The listing builds one solid part. Answer for the finished solid, in the listing's coordinates (mm). A direction names the side the tool comes from. Round coordinates to 2 decimals unless told otherwise and drop trailing zeros. Write each loop counter-clockwise with the first axis right and the second up, starting at its lowest first coordinate (ties: lowest second). Pieces come first, ordered by that corner, then holes.
(1) For faces 1 (the face through (18, 5, -0.1)), 2 (the face through (18, 0.808, -1)), 3 (the face through (18, 26, -2.4)), determine the directions among +Z, -Z, +X, -X, +Y, -Y from which every point of the face is accessible in a straight line to the end or side of a thin tool.
(2) Each of these flat-tipped pins is pushed along its axis until it touches: pin 1 Ø1.2 at (x, z) = (16, -1.5) entering from -Y; pin 2 Ø1.6 at (x, y) = (17, 4.5) entering from +Z. Where does it stop, or does it pass through?
(3) Find the intervals of material crossed by probe 1 along Y at (x, z) = (14, -1); probe 2 along Z at (x, y) = (29, 6), in increasing order.
(4) A cutting plane is placed at A-A, the plane x = 24. Give the vertices of the cut face in (y, z), and give its area (3 significant figures).
from build123d import *

# Parameters (mm, degrees)
ESQUISSE6_W             = 35.7
ESQUISSE6_H             = 51.2
BOSS_EXTRU_3_DEPTH      = 2.4
ESQUISSE7_W             = 33.59337029
ESQUISSE7_H             = 41.85
ENL_V_MAT_EXTRU_4_DEPTH = 0.1
ESQUISSE8_W             = 6.352818378
ESQUISSE8_H             = 0.449413723
ENL_V_MAT_EXTRU_5_DEPTH = 0.1
ESQUISSE9_W             = 31.478034176
ESQUISSE9_H             = 39.75
BOSS_EXTRU_4_DEPTH      = 0.1
ESQUISSE10_W            = 33.373849312
ESQUISSE10_H            = 5.346626879
ENL_V_MAT_EXTRU_6_DEPTH = 0.1
ESQUISSE11_W            = 23.638967436
ESQUISSE11_H            = 0.807997654
ENL_V_MAT_EXTRU_7_DEPTH = 63.463509347


with BuildPart() as part:
    # Esquisse6 → Boss.-Extru.3 (new body)
    with BuildSketch(Plane.XY):
        with Locations((17.85, 25.6)):
            Rectangle(ESQUISSE6_W, ESQUISSE6_H)
    extrude(amount=-BOSS_EXTRU_3_DEPTH)

    # Esquisse7 → Enlèv. mat.-Extru.4 (cut)
    with BuildSketch(Plane.XY):
        with Locations((17.85, 29.225)):
            Rectangle(ESQUISSE7_W, ESQUISSE7_H)
    extrude(amount=-ENL_V_MAT_EXTRU_4_DEPTH, mode=Mode.SUBTRACT)

    # Esquisse8 → Enlèv. mat.-Extru.5 (cut)
    with BuildSketch(Plane.XY):
        with Locations((17.85, 50.374706862)):
            Rectangle(ESQUISSE8_W, ESQUISSE8_H)
    extrude(amount=-ENL_V_MAT_EXTRU_5_DEPTH, mode=Mode.SUBTRACT)

    # Esquisse9 → Boss.-Extru.4 (add)
    with BuildSketch(Plane.XY.offset(-0.1)):
        with Locations((17.85, 29.225)):
            Rectangle(ESQUISSE9_W, ESQUISSE9_H)
    extrude(amount=BOSS_EXTRU_4_DEPTH)

    # Esquisse10 → Enlèv. mat.-Extru.6 (cut)
    with BuildSketch(Plane.XY):
        with Locations((17.915693231, 4.94567387)):
            Rectangle(ESQUISSE10_W, ESQUISSE10_H)
    extrude(amount=-ENL_V_MAT_EXTRU_6_DEPTH, mode=Mode.SUBTRACT)

    # Esquisse11 → Enlèv. mat.-Extru.7 (cut, through all)
    with BuildSketch(Plane.XY):
        with Locations((17.85, 0.403998827)):
            Rectangle(ESQUISSE11_W, ESQUISSE11_H)
    extrude(amount=-ENL_V_MAT_EXTRU_7_DEPTH, mode=Mode.SUBTRACT)


solid = part.part
Solutions:
1. face 1: +Z
1. face 2: +Z, -Z, -Y
1. face 3: -Z, +X, -X, +Y, -Y
2. pin 1: stops at y = 0.81
2. pin 2: stops at z = -0.1
3. probe 1: y = 0.81 to 51.2
3. probe 2: z = -2.4 to -0.1
4. outline: (0.81, -2.4) - (51.2, -2.4) - (51.2, 0) - (50.15, 0) - (50.15, -0.1) - (49.1, -0.1) - (49.1, 0) - (9.35, 0) - (9.35, -0.1) - (8.3, -0.1) - (8.3, 0) - (7.62, 0) - (7.62, -0.1) - (2.27, -0.1) - (2.27, 0) - (0.81, 0) - close
4. area: 120 mm2
